For this review, use the dimensioned drawing (mm, ordinates from the lowest corner) and the shaded views. A direction names the side the tool comes from. Give positions to 0.01 mm unless a question says otherwise; leave off trailing zeros. Write each loop counter-clockwise with the first axis right and the second up, starting at its lowest first coordinate (ties: lowest second). Pieces come first, ordered by that corner, then holes. Notation, with made-up numbers: (-29, -24) -> (7, -24) arc R8 ccw to (7, -15) -> close; hole circle Ø4 at (74.25, 87). An arc over 180 degrees is marked (long way). Write each question's results on one line, items separated by ' | '. Start each with the question number.
(1) Clearance check with flat-ended pins moving along their axes: pin 1 (9.5 mm diameter, centred on x = 15, z = 15, fed in from +Y); pin 2 (3 mm diameter, centred on x = 8.5, z = 18, fed in from -Y); pin 3 (8 mm diameter, centred on x = 21.5, y = 6, fed in from +Z); pin 4 (1 mm diameter, centred on y = 16, z = 16, fed in from -X). State where each tip first meets the part, or that it passes through.
(2) To check wall thickness, follow probe 1 along Z at (x, y) = (15, 20.75); probe 2 along Z at (x, y) = (22, 19); probe 3 along Z at (x, y) = (11.5, 6). State the ranges of each line that lie inside material, in increasing order.
(3) Take a section at C-C (z = 12.25). State the section outline as (x, y) points, plus the area to 3 significant figures.
(4) For the marked faces 1, 2 and 3, list the 3-axis set-ups (+Z, -Z, +X, -X, +Y, -Y) from which the entire face can be reached by the end or side of a thin tool; tool diameter is ignored.
(5) Take a section at A-A (z = 17.5). State the section outline as (x, y) points, plus the area to 3 significant figures.
(6) Take a section at B-B (z = 25.5). State the section outline as (x, y) points, plus the area to 3 significant figures.
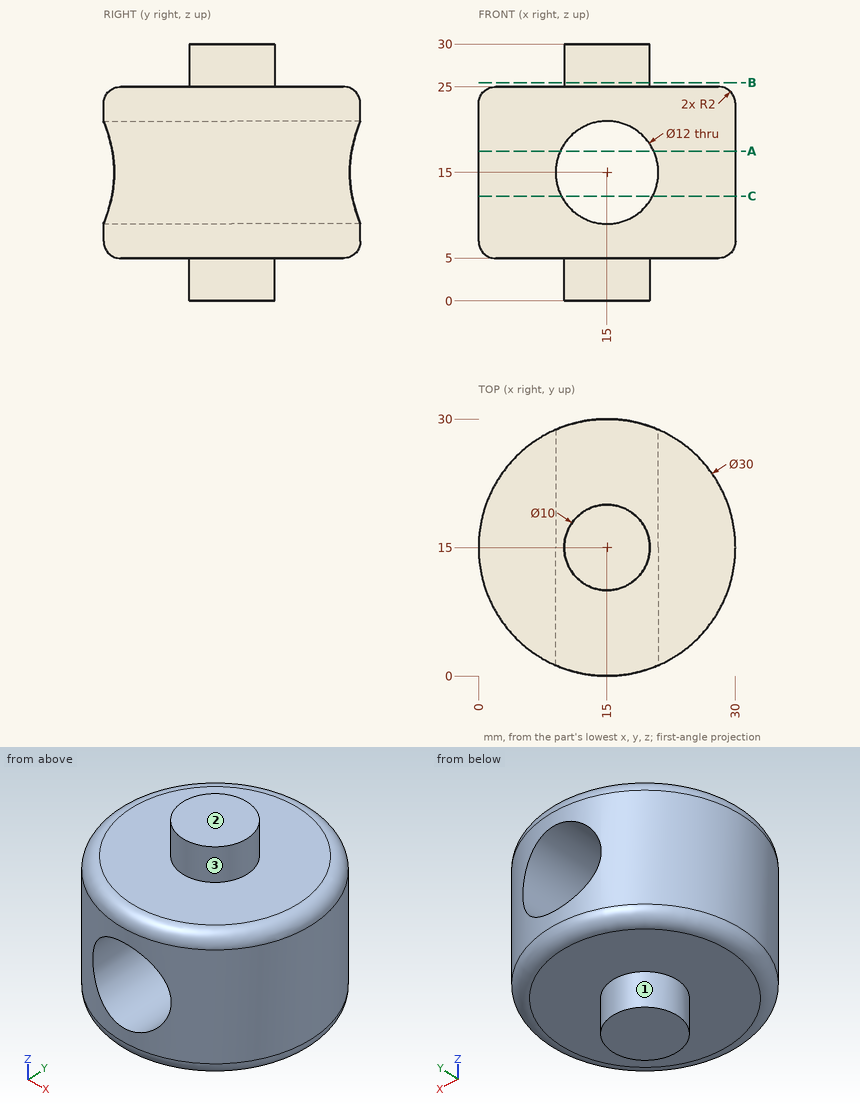
Report:
1) pin 1: through | pin 2: y = 0.87 | pin 3: z = 25 | pin 4: x = 0.01
2) probe 1: 5 to 9, 21 to 25 | probe 2: 5 to 25 | probe 3: 5 to 10.13, 19.87 to 25
3) outline: (9.67, 0.98) -> (9.67, 29.02) arc R15 ccw to start; (20.33, 0.98) arc R15 ccw to (20.33, 29.02) -> close | area: 394 mm2
4) face 1: -Z | face 2: +Z, +X, -X, +Y, -Y | face 3: +Z
5) outline: (9.55, 1.03) -> (9.55, 28.97) arc R15 ccw to start; (20.45, 1.03) arc R15 ccw to (20.45, 28.97) -> close | area: 387 mm2
6) outline: circle Ø10 at (15, 15) | area: 78.5 mm2
